Geometry check sheet. Reference: drawing and pictorial views, mm from the part's lowest x, y, z. Coordinates: 2 decimals unless noted, no trailing zeros. Loops run counter-clockwise (first coordinate to the right, second up) from the corner with the lowest first, then second, coordinate; pieces in that order, holes last. Notation, with made-up numbers: (51.5, 76) - (73.5, 76) arc R26 ccw to (73.5, 103) - close; hole circle Ø2 at (40, 89). An arc over 180 degrees is marked (long way). Use a Markdown table: item, result. Add a question column.
1) Sectioned sample at B-B, the plane z = 8.25. Enter the section's corners in (x, y), then the cut area to 3 significant figures.
2) Thickness scan on line 1 (Y direction, x = 6, z = 7.75); line 2 (X direction, y = 7.5, z = 7.75); line 3 (X direction, y = 9.5, z = 6.25). Record the ranges inside material, lowest first.
3) Go/stop test with a flat-tipped pin: P1, Ø10, axis at x = 37, y = 7.5, coming from the -Z side. Record where the tip stops, or that it passes through.
4) Sectioned sample at A-A, the plane x = 94. Enter the section's corners in (y, z), then the cut area to 3 significant figures.
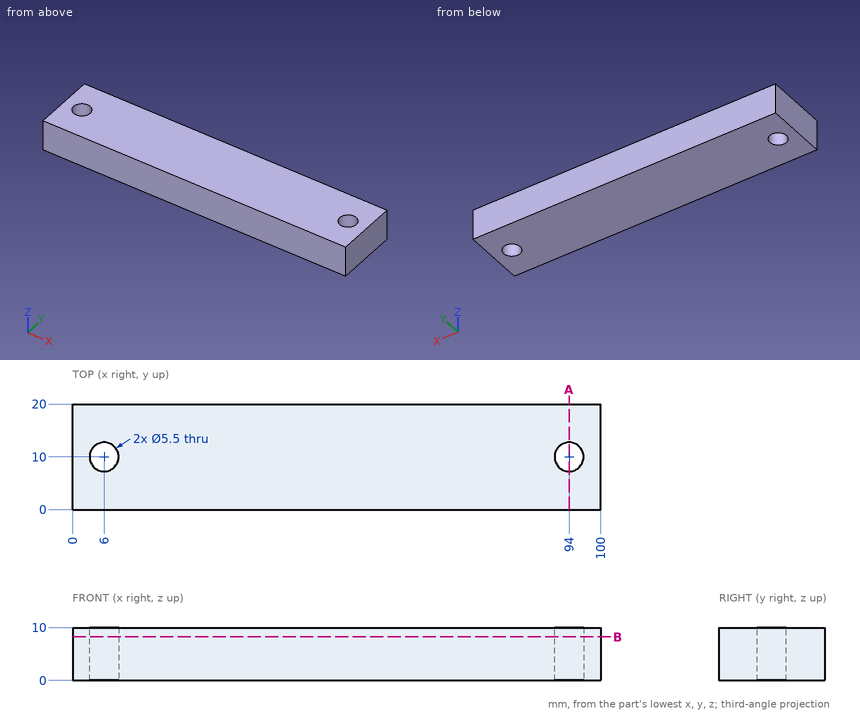
Solved:
| question | item | result |
|---|---|---|
| 1 | outline | (0, 0) - (100, 0) - (100, 20) - (0, 20) - close; hole circle Ø5.5 at (6, 10); hole circle Ø5.5 at (94, 10) |
| 1 | area | 1,950 mm2 |
| 2 | line 1 | y = 0 to 7.25, 12.75 to 20 |
| 2 | line 2 | x = 0 to 4.85, 7.15 to 92.85, 95.15 to 100 |
| 2 | line 3 | x = 0 to 3.3, 8.7 to 91.3, 96.7 to 100 |
| 3 | P1 | stops at z = 0 |
| 4 | outline | (0, 0) - (7.25, 0) - (7.25, 10) - (0, 10) - close; (12.75, 0) - (20, 0) - (20, 10) - (12.75, 10) - close |
| 4 | area | 145 mm2 |
